Check sheet for the modelled part. Datum: model origin and axes. Units: mm. Face numbers are marked on the shaded views. Coordinates: 2 decimals unless noted, no trailing zeros. Write each loop counter-clockwise with the first axis right and the second up, starting at its lowest first coordinate (ties: lowest second). Pieces come first, ordered by that corner, then holes. Notation, with made-up numbers: (13.5, -30.5) -> (17.5, -30.5) arc R28 ccw to (17.5, -7.5) -> close; hole circle Ø11 at (-32, 20). An arc over 180 degrees is marked (long way). Put each result on its own line as item: value.
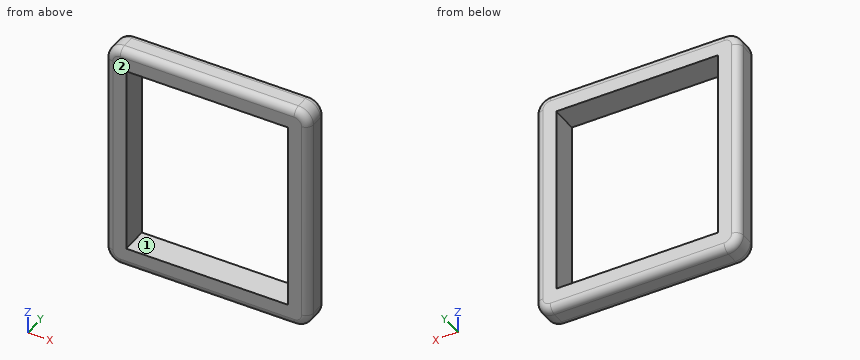
```python
from build123d import *

# Parameters (mm, degrees)
BOSS_EXTRUDE1_START = 38.1
SKETCH2_W           = 736.6
SKETCH2_H           = 863.6
SKETCH2_W_2         = 685.8
SKETCH2_H_2         = 812.8
BOSS_EXTRUDE1_DEPTH = 114.3


with BuildPart() as part:
    # Sketch2 → Boss-Extrude1 (new body)
    with BuildSketch(Plane(origin=(0, 0, 0), x_dir=(1, 0, 0), z_dir=(0, 1, 0)).offset(BOSS_EXTRUDE1_START)):
        Rectangle(SKETCH2_W, SKETCH2_H)
        Rectangle(SKETCH2_W_2, SKETCH2_H_2, mode=Mode.SUBTRACT)
    extrude(amount=BOSS_EXTRUDE1_DEPTH)

    # Sweep1: sweep along a path in Sketch4
    with BuildLine(Plane(origin=(0, 152.4, 0), x_dir=(1, 0, 0), z_dir=(0, 1, 0))) as sweep1_path:
        Line((368.3, 495.3), (-368.3, 495.3))
        ThreePointArc((-368.3, 495.3), (-413.201280605, 476.701280605), (-431.8, 431.8))
        Line((-431.8, 431.8), (-431.8, -431.8))
        ThreePointArc((-431.8, -431.8), (-413.201280605, -476.701280605), (-368.3, -495.3))
        Line((-368.3, -495.3), (368.3, -495.3))
        ThreePointArc((368.3, -495.3), (413.201280605, -476.701280605), (431.8, -431.8))
        Line((431.8, -431.8), (431.8, 431.8))
        ThreePointArc((431.8, 431.8), (413.201280605, 476.701280605), (368.3, 495.3))
    # Sketch3 → Sweep1 (sweep)
    with BuildSketch(Plane.XY.offset(431.8)):
        with BuildLine():
            Line((-400.05, 152.4), (-368.3, 152.4))
            Line((-368.3, 152.4), (-368.3, 38.1))
            Line((-368.3, 38.1), (-400.05, 38.1))
            ThreePointArc((-400.05, 38.1), (-422.500640303, 47.399359697), (-431.8, 69.85))
            Line((-431.8, 69.85), (-431.8, 120.65))
            ThreePointArc((-431.8, 120.65), (-422.500640303, 143.100640303), (-400.05, 152.4))
        make_face()
    sweep(path=sweep1_path.line)


solid = part.part
```
Q1. Material ranges on line 1 along X through (y, z) = (75.5, 284); line 2 along Z through (x, y) = (-205.5, 113); line 3 along X through (y, z) = (123, 341.5), recorded low to high.
Recorded:
line 1: x = -431.8 to -342.9, 342.9 to 431.8
line 2: z = -495.3 to -406.4, 406.4 to 495.3
line 3: x = -431.71 to -342.9, 342.9 to 431.71
Q2. Cross-section at B-B (x = 154). Record the cut outline in (y, z), plus the area to 3 significant figures.
Recorded:
outline: (38.1, -463.55) arc R31.75 ccw to (69.85, -495.3) -> (120.65, -495.3) arc R31.75 ccw to (152.4, -463.55) -> (152.4, -406.4) -> (38.1, -406.4) -> close; (38.1, 406.4) -> (152.4, 406.4) -> (152.4, 463.55) arc R31.75 ccw to (120.65, 495.3) -> (69.85, 495.3) arc R31.75 ccw to (38.1, 463.55) -> close
area: 19,500 mm2
Q3. Depth check by flat-ended pin: P1, Ø10, axis at y = 63, z = -124.5, coming from the +X side; P2, Ø1.5, axis at y = 61.5, z = 94, coming from the -X side; P3, Ø4, axis at y = 64.5, z = -276, coming from the -X side. Enter the tip coordinate at first touch or a pass-through.
Recorded:
P1: stops at x = 431.75
P2: stops at x = -430.88
P3: stops at x = -431.62
Q4. Cross-section at A-A (y = 84). Record the cut outline in (x, z), plus the area to 3 significant figures.
Recorded:
outline: (-431.8, -431.8) arc R63.5 ccw to (-368.3, -495.3) -> (368.3, -495.3) arc R63.5 ccw to (431.8, -431.8) -> (431.8, 431.8) arc R63.5 ccw to (368.3, 495.3) -> (-368.3, 495.3) arc R63.5 ccw to (-431.8, 431.8) -> close; hole (-342.9, -406.4) -> (342.9, -406.4) -> (342.9, 406.4) -> (-342.9, 406.4) -> close
area: 295,000 mm2
Q5. Mould release check, pull along Z, two halves, no side actions. Record for the marked faces 1 and 2: released by +Z, released by -Z, zero draft, split by the parting line, or undercut.
Recorded:
face 1: undercut
face 2: zero draft
